Verification items for this drawing (mm, ordinates from the low corner). A direction names the side the tool comes from. Give positions to 0.01 mm unless a question says otherwise; leave off trailing zeros. Loops run counter-clockwise (first coordinate to the right, second up) from the corner with the lowest first, then second, coordinate; pieces in that order, holes last. Notation, with made-up numbers: M 82.5,28.25 L 107.5,28.25 A12 cw 107.5,32.25 Z; hole C 41,23.5 d10. An arc over 180 degrees is marked long. Put each result on its own line as item: value. Start each with the question number.
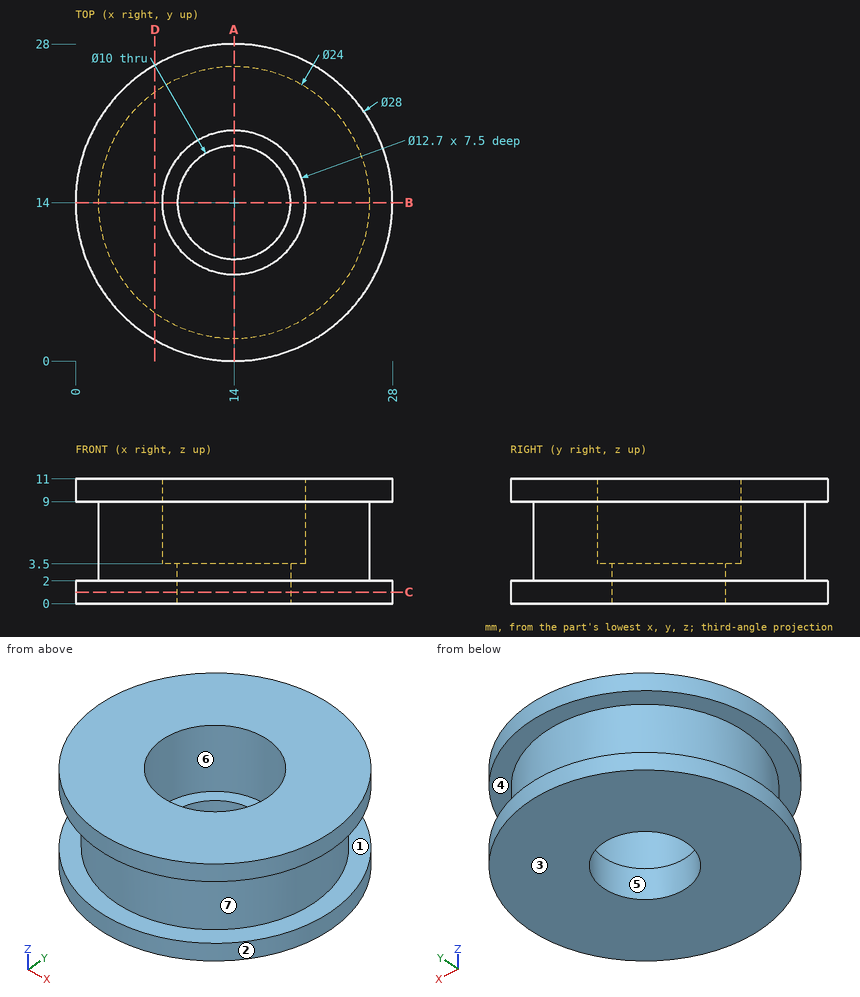
Q1. Cross-section at C-C, the plane z = 1. Record the boundary of the cut face in (x, y), then the cut area to 3 significant figures.
Q2. Scan lines: L1, parallel to Z at x = 1.5, y = 20; L2, parallel to Y at x = 14, z = 7.75; L3, parallel to Y at x = 14, z = 1.4. Record each from-to range of solid material in increasing order.
Q3. Cross-section at A-A, the plane x = 14. Record the boundary of the cut face in (y, z), then the cut area to 3 significant figures.
Q4. Go/stop test with flat-tipped pins: pin 1 (10 mm diameter, centred on x = 13.5, y = 13.5, fed in from +Z); pin 2 (5 mm diameter, centred on x = 19.5, z = 7.5, fed in from +Y). Record where each tip stops, or that it passes through.
Q5. Cross-section at D-D, the plane x = 7. Record the boundary of the cut face in (y, z).
Q6. Release check for a two-part mould opening along Z. For the marked faces 1, 2, 3 and 4 record: pulls with the +Z half, pulls with the -Z half, needs draft (parallel to the pull), parting line crosses it, or undercut.
Q7. Set-up check for the marked faces 5, 6 and 7: record each of +Z, -Z, +X, -X, +Y, -Y from which the full face is reachable in a straight line by a thin tool's end or side.
Ans:
1. outline: C 14,14 d28; hole C 14,14 d10
1. area: 537 mm^2
2. L1: z = 0 to 2, 9 to 11
2. L2: y = 2 to 7.65, 20.35 to 26
2. L3: y = 0 to 9, 19 to 28
3. outline: M 0,0 L 9,0 L 9,3.5 L 7.65,3.5 L 7.65,11 L 0,11 L 0,9 L 2,9 L 2,2 L 0,2 Z; M 19,0 L 28,0 L 28,2 L 26,2 L 26,9 L 28,9 L 28,11 L 20.35,11 L 20.35,3.5 L 19,3.5 Z
3. area: 150 mm^2
4. pin 1: stops at z = 3.5
4. pin 2: stops at y = 27.56
5. outline: M 1.88,0 L 26.12,0 L 26.12,2 L 23.75,2 L 23.75,9 L 26.12,9 L 26.12,11 L 1.88,11 L 1.88,9 L 4.25,9 L 4.25,2 L 1.88,2 Z
6. face 1: undercut
6. face 2: needs draft
6. face 3: pulls with the -Z half
6. face 4: undercut
7. face 5: +Z, -Z
7. face 6: +Z
7. face 7: none
